from build123d import *

# Parameters (mm, degrees)
SKETCH001_W     = 99
SKETCH001_H     = 81
PAD001_DEPTH    = 15
THICKNESS001_T  = 3
SKETCH003_R     = 1.6
POCKET001_DEPTH = 12.001
SKETCH005_W     = 24
SKETCH005_H     = 25
POCKET002_DEPTH = 18.001
SKETCH006_W     = 15
SKETCH006_H     = 8
POCKET003_DEPTH = 3
SKETCH007_W     = 17
SKETCH007_H     = 6.5
POCKET004_DEPTH = 3
SKETCH008_W     = 20
SKETCH008_H     = 8
POCKET005_DEPTH = 3
SKETCH009_W     = 22
SKETCH009_H     = 10
POCKET006_DEPTH = 3
SKETCH010_W     = 2
SKETCH010_H     = 3.5
SKETCH010_W_2   = 12.528473
SKETCH010_H_2   = 2
SKETCH010_W_3   = 9.705046
SKETCH010_W_4   = 7.019181
SKETCH010_W_5   = 13.364327
SKETCH010_W_6   = 7.581009
POCKET007_DEPTH = 3
SKETCH011_R     = 1.5
PAD002_DEPTH    = 7


with BuildPart() as part:
    # Sketch001 → Pad001 (new body)
    with BuildSketch(Plane.XY.offset(25)):
        with Locations((20, -91.5)):
            Rectangle(SKETCH001_W, SKETCH001_H)
    extrude(amount=PAD001_DEPTH)

    # Thickness001
    thickness001_openings = [part.faces().sort_by_distance(p)[0] for p in [
        (20, -91.5, 25),
    ]]
    offset(amount=THICKNESS001_T, openings=thickness001_openings)

    # Sketch003 (on Part__Feature) → Pocket001 (cut, through all)
    with BuildSketch(Plane(origin=(-200, 0, 37), x_dir=(1, 0, 0), z_dir=(0, 0, 1))):
        with Locations((180, -63)):
            Circle(SKETCH003_R)
        with Locations((254, -124)):
            Circle(SKETCH003_R)
    extrude(amount=-POCKET001_DEPTH, mode=Mode.SUBTRACT)

    # Sketch005 (on Face23 of Pocket001) → Pocket002 (cut, through all)
    with BuildSketch(Plane.XY.offset(43)):
        with Locations((52.5, -90.5)):
            Rectangle(SKETCH005_W, SKETCH005_H)
    extrude(amount=-POCKET002_DEPTH, mode=Mode.SUBTRACT)

    # Sketch006 (on Face10 of Pocket002) → Pocket003 (cut)
    with BuildSketch(Plane(origin=(-32.5, 0, 0), x_dir=(0, -1, 0), z_dir=(-1, 0, 0))):
        with Locations((97.5, 30)):
            Rectangle(SKETCH006_W, SKETCH006_H)
    extrude(amount=-POCKET003_DEPTH, mode=Mode.SUBTRACT)

    # Sketch007 (on Face12 of Pocket003) → Pocket004 (cut)
    with BuildSketch(Plane(origin=(0, -48, 0), x_dir=(-1, 0, 0), z_dir=(0, 1, 0))):
        with Locations((6, 29.75)):
            Rectangle(SKETCH007_W, SKETCH007_H)
    extrude(amount=-POCKET004_DEPTH, mode=Mode.SUBTRACT)

    # Sketch008 (on Face22 of Pocket004) → Pocket005 (cut)
    with BuildSketch(Plane.YZ.offset(72.5)):
        with Locations((-116, 30.5)):
            Rectangle(SKETCH008_W, SKETCH008_H)
    extrude(amount=-POCKET005_DEPTH, mode=Mode.SUBTRACT)

    # Sketch009 (on Face20 of Pocket005) → Pocket006 (cut)
    with BuildSketch(Plane.XZ.offset(135)):
        with Locations((23.5, 33)):
            Rectangle(SKETCH009_W, SKETCH009_H)
    extrude(amount=-POCKET006_DEPTH, mode=Mode.SUBTRACT)

    # Sketch010 (on Face43 of Pocket006) → Pocket007 (cut)
    with BuildSketch(Plane.XY.offset(43)):
        with Locations((-9.15269, -80.468796)):
            Rectangle(SKETCH010_W, SKETCH010_H)
        with Locations((-3.888453, -77.718796)):
            Rectangle(SKETCH010_W_2, SKETCH010_H_2)
        with Locations((-3.888453, -83.218796)):
            Rectangle(SKETCH010_W_2, SKETCH010_H_2)
        with Locations((-0.087345, -89.722328)):
            Rectangle(SKETCH010_W, SKETCH010_H)
        with Locations((3.765178, -86.972328)):
            Rectangle(SKETCH010_W_3, SKETCH010_H_2)
        with Locations((3.765178, -92.472328)):
            Rectangle(SKETCH010_W_3, SKETCH010_H_2)
        with Locations((-8.900494, -89.722328)):
            Rectangle(SKETCH010_W, SKETCH010_H)
        with Locations((-6.390904, -86.972328)):
            Rectangle(SKETCH010_W_4, SKETCH010_H_2)
        with Locations((-6.390904, -92.472328)):
            Rectangle(SKETCH010_W_4, SKETCH010_H_2)
        with Locations((-9.392209, -98.730659)):
            Rectangle(SKETCH010_W, SKETCH010_H)
        with Locations((-3.710045, -95.980659)):
            Rectangle(SKETCH010_W_5, SKETCH010_H_2)
        with Locations((-3.710045, -101.480659)):
            Rectangle(SKETCH010_W_5, SKETCH010_H_2)
        with Locations((-18.626614, -89.722328)):
            Rectangle(SKETCH010_W, SKETCH010_H)
        with Locations((-15.836109, -86.972328)):
            Rectangle(SKETCH010_W_6, SKETCH010_H_2)
        with Locations((-15.836109, -92.472328)):
            Rectangle(SKETCH010_W_6, SKETCH010_H_2)
    extrude(amount=-POCKET007_DEPTH, mode=Mode.SUBTRACT)

    # Sketch011 (on Face4 of Pocket007) → Pad002 (join)
    with BuildSketch(Plane(origin=(0, 0, 40), x_dir=(1, 0, 0), z_dir=(0, 0, -1))):
        with Locations((-6.596659, 98.725481)):
            Circle(SKETCH011_R)
        with Locations((2.745978, 89.787056)):
            Circle(SKETCH011_R)
        with Locations((-6.275136, 89.713417)):
            Circle(SKETCH011_R)
        with Locations((-6.42242, 80.397736)):
            Circle(SKETCH011_R)
        with Locations((-16.017, 89.712753)):
            Circle(SKETCH011_R)
    extrude(amount=PAD002_DEPTH)


solid = part.part
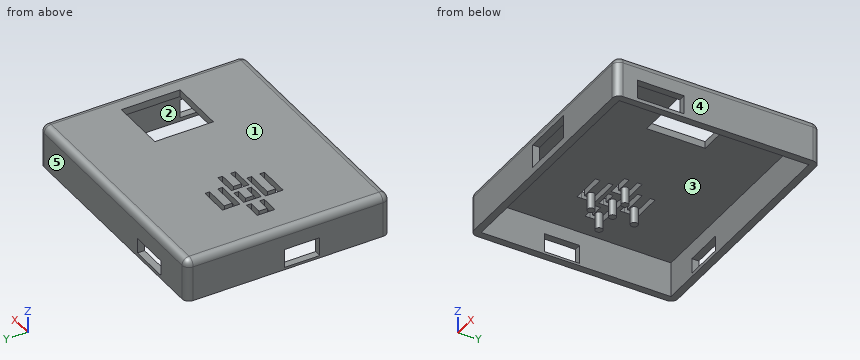
Read the model definition and answer for the solid it produces. Units are mm, in the model's axes. Face numbers are marked on the shaded views. A direction names the side the tool comes from. Coordinates: 2 decimals unless noted, no trailing zeros. Loops run counter-clockwise (first coordinate to the right, second up) from the corner with the lowest first, then second, coordinate; pieces in that order, holes last.
Q1. Consider probe 1 along Y at (x, z) = (51, 30); probe 2 along X at (y, z) = (-56.5, 32.5); probe 3 along X at (y, z) = (-91, 38.5). Determine where each line is inside the solid, lowest interval first.
Q2. Each of these flat-tipped pins is pushed along its axis until it touches: pin 1 Ø1 at (y, z) = (-101.5, 42) entering from +X; pin 2 Ø2 at (y, z) = (-87.5, 41) entering from -X; pin 3 Ø1.6 at (y, z) = (-92, 42) entering from -X; pin 4 Ø4 at (x, y) = (37, -119) entering from -Z. Where does it stop, or does it pass through?
Q3. The part is cut by section A-A on x = 31. Write down the section's boundary in (y, z).
Q4. The part is cut by section B-B on y = -65. Write down the section's boundary in (x, z).
Q5. The part is cut by section D-D on z = 41.5. Give the number of separate pieces and of enclosed holes in the cut face, and give its area (3 significant figures).
Q6. The part is cut by section C-C on x = 58. Write down the section's boundary in (y, z).
Q7. The mould has two halves that part along Y. Classify the marked faces 3, 4 and 5: +Y half, -Y half, draft (parallel to the pull), parting line (faces both ways), or undercut.
Q8. Which of the six approach directions +Z, -Z, +X, -X, +Y, -Y give full straight-line access (tool end or side, diameter ignored) to the marked faces 1 and 2?
Results below:
1. probe 1: y = -135 to -132, -51 to -48
1. probe 2: x = -32.5 to -29.5, 69.5 to 72.5
1. probe 3: x = -32.5 to -29.5, -16.79 to -15.25, -7.05 to -5.5, 1.86 to 3.63, 69.5 to 72.5
2. pin 1: stops at x = 72.1
2. pin 2: stops at x = -32.5
2. pin 3: stops at x = -32.25
2. pin 4: stops at z = 40
3. outline: (-135, 25) - (-132, 25) - (-132, 28) - (-135, 28) - close; (-135, 38) - (-132, 38) - (-132, 40) - (-51, 40) - (-51, 25) - (-48, 25) - (-48, 40) arc R3 ccw to (-51, 43) - (-132, 43) arc R3 ccw to (-135, 40) - close
4. outline: (-32.5, 25) - (-29.5, 25) - (-29.5, 40) - (69.5, 40) - (69.5, 25) - (72.5, 25) - (72.5, 40) arc R3 ccw to (69.5, 43) - (-29.5, 43) arc R3 ccw to (-32.5, 40) - close
5. separate pieces: 1
5. enclosed holes: 6
5. area: 8,140 mm2
6. outline: (-135, 25) - (-132, 25) - (-132, 40) - (-103, 40) - (-103, 43) - (-132, 43) arc R3 ccw to (-135, 40) - close; (-78, 40) - (-51, 40) - (-51, 25) - (-48, 25) - (-48, 40) arc R3 ccw to (-51, 43) - (-78, 43) - close
7. face 3: undercut
7. face 4: draft
7. face 5: +Y half
8. face 1: +Z, +X, -X, +Y, -Y
8. face 2: -Z
